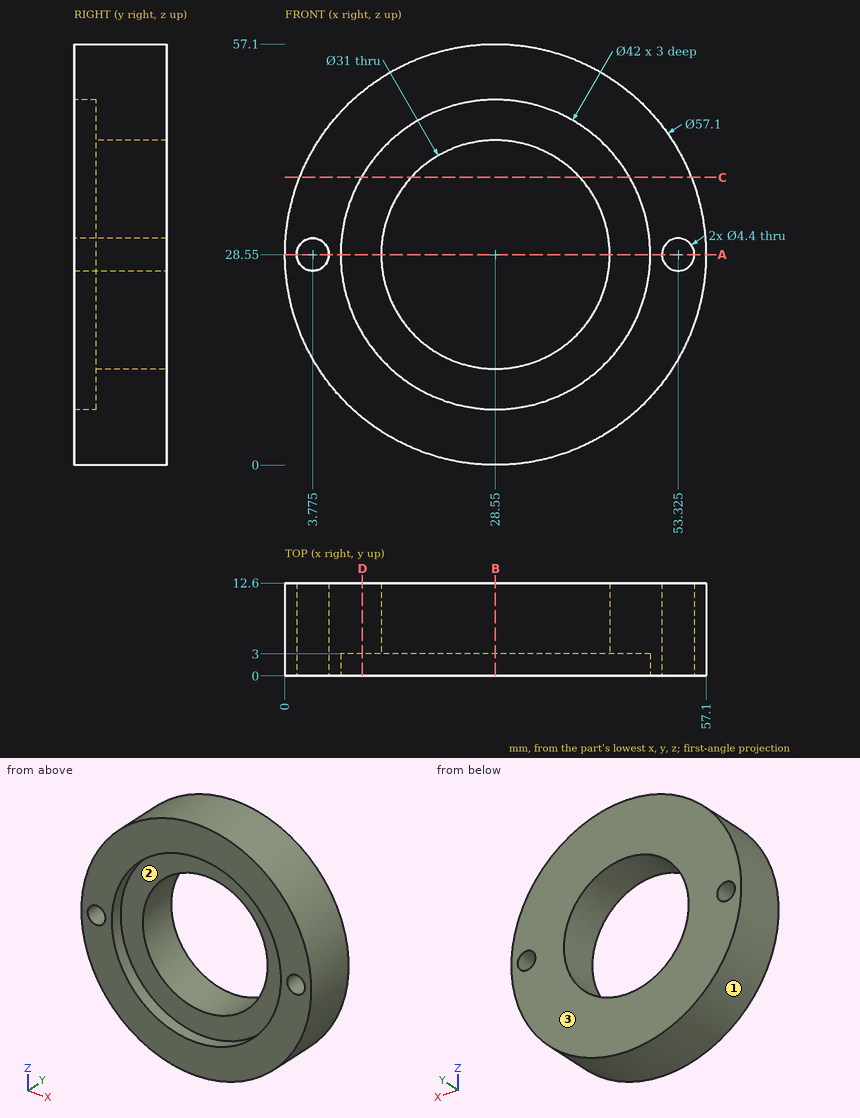
Can you work these out from the drawing? Everything is in mm from the part's minimum corner. Give positions to 0.01 mm unless a question says otherwise; leave off trailing zeros. Order: outer loops, then holes, each group sorted by start corner. A loop starts at its lowest first (then second) coordinate and runs counter-clockwise, first axis right, second up.
Item 1: I need wall thicknesses on line 1 (X direction, y = 8, z = 28.55) (3 decimals); line 2 (Y direction, x = 20, z = 47); line 3 (X direction, y = 3.75, z = 37). Which ranges of each line are inside material? Lowest first, please.
Item 2: I'm going to push flat-ended pins straight in: pin 1 (2 mm diameter, centred on x = 33, y = 8, fed in from -Z); pin 2 (4 mm diameter, centred on y = 4.5, z = 10, fed in from -X); pin 3 (2 mm diameter, centred on y = 10.5, z = 44, fed in from -X); pin 4 (3.5 mm diameter, centred on x = 53.325, z = 28.55, fed in from -Y). Where does each tip first touch, or does it pass through?
Item 3: If we section it at A-A, the plane z = 28.55: Write out the boundary of the cut face in (x, y) (3 decimals), plus the area to 3 significant figures.
Item 4: If we section it at D-D, the plane x = 10.5: Write out the boundary of the cut face in (y, z), plus the area to 3 significant figures.
Item 5: If we mould it in two halves opening along X, with no side actions, what happens to the marked faces 1, 2 and 3? For each: pulls with the +X half, pulls with the -X half, needs draft (parallel to the pull), parting line crosses it, or undercut.
Item 6: If we section it at C-C, the plane z = 39: Write out the boundary of the cut face in (x, y), plus the area to 3 significant figures.
Item 7: If we section it at B-B, the plane x = 28.55: Write out the boundary of the cut face in (y, z).
Values:
1. line 1: x = 0 to 1.575, 5.975 to 13.05, 44.05 to 51.125, 55.525 to 57.1
1. line 2: y = 3 to 12.6
1. line 3: x = 1.28 to 15.56, 41.54 to 55.82
2. pin 1: stops at z = 0.21
2. pin 2: stops at x = 5.29
2. pin 3: stops at x = 3.93
2. pin 4: passes through
3. outline: (0, 0) - (1.575, 0) - (1.575, 12.6) - (0, 12.6) - close; (5.975, 0) - (7.55, 0) - (7.55, 3) - (13.05, 3) - (13.05, 12.6) - (5.975, 12.6) - close; (44.05, 3) - (49.55, 3) - (49.55, 0) - (51.125, 0) - (51.125, 12.6) - (44.05, 12.6) - close; (55.525, 0) - (57.1, 0) - (57.1, 12.6) - (55.525, 12.6) - close
3. area: 185 mm2
4. outline: (0, 6.43) - (12.6, 6.43) - (12.6, 50.67) - (0, 50.67) - (0, 39.28) - (3, 39.28) - (3, 17.82) - (0, 17.82) - close
4. area: 493 mm2
5. face 1: parting line crosses it
5. face 2: undercut
5. face 3: needs draft
6. outline: (1.98, 0) - (10.33, 0) - (10.33, 3) - (17.1, 3) - (17.1, 12.6) - (1.98, 12.6) - close; (40, 3) - (46.77, 3) - (46.77, 0) - (55.12, 0) - (55.12, 12.6) - (40, 12.6) - close
6. area: 340 mm2
7. outline: (0, 0) - (12.6, 0) - (12.6, 13.05) - (3, 13.05) - (3, 7.55) - (0, 7.55) - close; (0, 49.55) - (3, 49.55) - (3, 44.05) - (12.6, 44.05) - (12.6, 57.1) - (0, 57.1) - close
